```python
from build123d import *

# Parameters (mm, degrees)
BOSS_EXTRUDE1_DEPTH          = 3.175
F_10_0_1935_DIAMETER_HOLE2_D = 4.9149
SKETCH5_R                    = 2.5527
SKETCH5_R_2                  = 14.2875
CUT_EXTRUDE2_DEPTH           = 6.35


with BuildPart() as part:
    # Sketch2 → Boss-Extrude1 (new body)
    with BuildSketch(Plane.XY):
        Polygon((0, 63.5), (-1.5875, 63.5), (-1.5875, 30.1625), (0, 30.1625), (0, 0), (30.1625, 0), (30.1625, -1.5875), (547.6875, -1.5875), (547.6875, 0), (577.85, 0), (577.85, 30.1625), (579.4375, 30.1625), (579.4375, 63.5), (577.85, 63.5), (577.85, 93.6625), (547.6875, 93.6625), (547.6875, 95.25), (30.1625, 95.25), (30.1625, 93.6625), (0, 93.6625), align=None)
    extrude(amount=BOSS_EXTRUDE1_DEPTH)

    # #10 (0.1935) Diameter Hole2 (through all)
    with Locations(Plane.XY.offset(3.175)):
        with Locations((288.925, 79.375), (123.825, 79.375), (454.025, 79.375), (454.025, 14.2875), (123.825, 14.2875), (288.925, 14.2875)):
            Hole(F_10_0_1935_DIAMETER_HOLE2_D / 2)

    # Sketch5 → Cut-Extrude2 (cut)
    with BuildSketch(Plane(origin=(0, 0, 0), x_dir=(-1, 0, 0), z_dir=(0, 0, -1))):
        with Locations((-541.825524484, 40.195494446)):
            Circle(SKETCH5_R)
        with Locations((-505.92448107, 4.2545)):
            Circle(SKETCH5_R)
        with Locations((-523.875002777, 22.224997223)):
            Circle(SKETCH5_R_2)
        with Locations((-541.8455, 4.274475516)):
            Circle(SKETCH5_R)
        with Locations((-505.904505554, 40.17551893)):
            Circle(SKETCH5_R)
        with Locations((-71.945494446, 40.17551893)):
            Circle(SKETCH5_R)
        with Locations((-36.0045, 4.274475516)):
            Circle(SKETCH5_R)
        with Locations((-53.974997223, 22.224997223)):
            Circle(SKETCH5_R_2)
        with Locations((-71.92551893, 4.2545)):
            Circle(SKETCH5_R)
        with Locations((-36.024475516, 40.195494446)):
            Circle(SKETCH5_R)
    extrude(amount=-CUT_EXTRUDE2_DEPTH, mode=Mode.SUBTRACT)


solid = part.part
```
Source: CAD feature listing. Evaluate the final solid. Frame: model axes, mm. Give positions to 0.01 mm unless a question says otherwise; leave off trailing zeros.
(1) Contact query for flat-ended pins moving along their axis: P1, Ø4.5, axis at x = 71.95, y = 40.18, coming from the -Z side; P2, Ø1.6, axis at y = 84.5, z = 1.5, coming from the -X side; P3, Ø0.8, axis at x = -0.5, z = 2, coming from the +Y side; P4, Ø1.6, axis at x = 567, z = 2, coming from the -Y side. Output: stop coordinate, or through.
(2) Pull-direction query (X, two-part tool) for faces 1 (the face through (510.68, 16.75, 1.57)), 2 (the face through (47.38, 9.55, 1.57)), 3 (the face through (285, 48, 3.175)); classes: +X half, -X half, draft (parallel to the pull), parting line (faces both ways), or undercut.
(3) Section query A-A (z = 1.05). State how many separate pieces and enclosed holes the cut face has, plus the area to 3 significant figures.
(4) Material intervals for line 1 along X through (y, z) = (17, 2.65); line 2 along X through (y, z) = (12.5, 0.95); line 3 along X through (y, z) = (34, 1.65), sorted ascending.
Outcome:
1. P1: passes through
1. P2: stops at x = 0
1. P3: stops at y = 63.5
1. P4: stops at y = 0
2. face 1: undercut
2. face 2: undercut
2. face 3: draft
3. separate pieces: 1
3. enclosed holes: 16
3. area: 54,300 mm2
4. line 1: x = 0 to 40.68, 67.27 to 510.58, 537.17 to 577.85
4. line 2: x = 0 to 43.51, 64.44 to 122.14, 125.51 to 287.24, 290.61 to 452.34, 455.71 to 513.41, 534.34 to 577.85
4. line 3: x = -1.59 to 45.88, 62.07 to 515.78, 531.97 to 579.44
